Geometry: final body of the model. Coordinates: model frame, mm. Face numbers are marked on the shaded views. A direction names the side the tool comes from. Coordinates: 2 decimals unless noted, no trailing zeros. Order: outer loops, then holes, each group sorted by start corner. A loop starts at its lowest first (then second) coordinate and runs counter-clockwise, first axis right, second up. Notation, with made-up numbers: (56, -17) -> (90, -17) arc R12 ccw to (90, 4) -> close; hole circle Ø4 at (11.5, 51). An arc over 180 degrees is marked (long way). Use one line per item in the form item = value.
Autodesk Inventor part; units mm, degrees
ref_plane "YZ Plane" through (0, 0, 0) normal (1, 0, 0) x (0, 1, 0)
ref_plane "XZ Plane" through (0, 0, 0) normal (0, 1, 0) x (-1, 0, 0)
ref_plane "XY Plane" through (0, 0, 0) normal (0, 0, 1) x (1, 0, 0)
sketch "Sketch1" plane through (0, 0, 0) normal (0, 1, 0) x (-1, 0, 0)
  line L0 (0, 0) -> (30, 0) construction
  line L1 (30, 0) -> (30, -6) construction
  line L2 (30, -6) -> (30, -13)
  line L3 (0, -87.5) -> (20, -87.5)
  line L4 (20, -87.5) -> (20, -67.5)
  line L5 (30, -6) -> (0, -6)
  line L6 (0, 0) -> (0, -87.5) construction
  line L7 (0, 0) -> (-30, 0) construction
  line L8 (-30, 0) -> (-30, -6) construction
  line L9 (-30, -6) -> (-30, -13)
  line L10 (0, -87.5) -> (-20, -87.5)
  line L11 (-20, -87.5) -> (-20, -67.5)
  line L12 (-30, -6) -> (0, -6)
  line L13 (20, -67.5) -> (10, -67.5)
  line L14 (10, -67.5) -> (10, -13)
  line L15 (10, -13) -> (30, -13)
  line L16 (-10, -67.5) -> (-10, -13)
  line L17 (-10, -13) -> (-30, -13)
  line L18 (-20, -67.5) -> (-10, -67.5)
  dimension "d0" = 30
  dimension "d1" = 6
  dimension "d3" = 7
  dimension "d4" = 20
  dimension "d5" = 87.5
  dimension "d6" = 20
  dimension "d8" = 10
revolve "Revolution1" add sketch "Sketch1" angle 360 about axis through (0, 0, 0) along (1, 0, 0)
properties part number "PK"
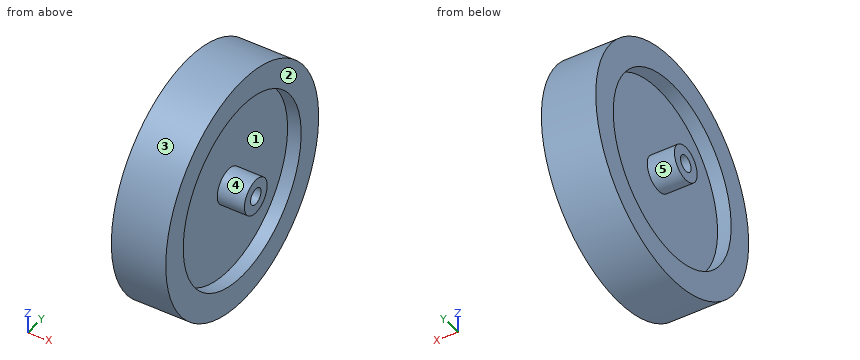
1) Access query for the marked faces 4 and 5. Directions: +Z, -Z, +X, -X, +Y, -Y. A direction counts if a zero-diameter tool reaches every point of the face in a straight line with its end or side. Return the directions, or none.
Results found:
face_4 = +X
face_5 = -X
2) Contact query for flat-ended pins moving along their axis: P1, Ø2, axis at x = -14, z = 22.5, coming from the +Y side; P2, Ø2, axis at x = 0, y = -16.5, coming from the -Z side; P3, Ø1, axis at y = -2.5, z = 62, coming from the +X side. Output: stop coordinate, or through.
Results found:
P1 = 84.82
P2 = -86.12
P3 = 10
3) Material intervals for probe 1 along Y at (x, z) = (-14, 0); probe 2 along Y at (x, z) = (11.5, 8); probe 3 along Y at (x, z) = (-6, 0), sorted ascending. Write a range as from..to.
Results found:
probe_1 = -87.5..-67.5, -13..-6, 6..13, 67.5..87.5
probe_2 = -87.13..-67.02, -10.25..10.25, 67.02..87.13
probe_3 = -87.5..-6, 6..87.5
4) Section D-D, the plane y = -22. Output: boundary loops of the cut face in (x, z).
Results found:
outline = (-20, -84.69) -> (20, -84.69) -> (20, -63.81) -> (10, -63.81) -> (10, 63.81) -> (20, 63.81) -> (20, 84.69) -> (-20, 84.69) -> (-20, 63.81) -> (-10, 63.81) -> (-10, -63.81) -> (-20, -63.81) -> close
5) Pull-direction query (Y, two-part tool) for the marked faces 1, 2 and 3; classes: released by +Y, released by -Y, zero draft, split by the parting line, or undercut.
Results found:
face_1 = undercut
face_2 = zero draft
face_3 = split by the parting line
6) Section A-A, the plane y = 0. Output: boundary loops of the cut face in (x, z), and give its area (3 significant figures).
Results found:
outline = (-30, -13) -> (-10, -13) -> (-10, -67.5) -> (-20, -67.5) -> (-20, -87.5) -> (20, -87.5) -> (20, -67.5) -> (10, -67.5) -> (10, -13) -> (30, -13) -> (30, -6) -> (-30, -6) -> close; (-30, 6) -> (30, 6) -> (30, 13) -> (10, 13) -> (10, 67.5) -> (20, 67.5) -> (20, 87.5) -> (-20, 87.5) -> (-20, 67.5) -> (-10, 67.5) -> (-10, 13) -> (-30, 13) -> close
area = 4,620 mm2
7) Section C-C, the plane x = -3. Output: boundary loops of the cut face in (y, z).
Results found:
outline = circle Ø175 at (0, 0); hole circle Ø12 at (0, 0)
